Check sheet for the modelled part. Datum: model origin and axes. Units: mm. Face numbers are marked on the shaded views. A direction names the side the tool comes from. Give positions to 0.01 mm unless a question says otherwise; leave off trailing zeros. Loops run counter-clockwise (first coordinate to the right, second up) from the corner with the lowest first, then second, coordinate; pieces in that order, holes last. Notation, with made-up numbers: M 25.25,3.25 L 54.25,3.25 A23 ccw 54.25,28.25 Z; hole C 52,67 d9. An arc over 180 degrees is marked long. One line per question, with ' | ' between items. Start each with the question number.
from build123d import *

# Parameters (mm, degrees)
BOSS_EXTRUDE1_DEPTH = 22
SKETCH3_R           = 26.2
CUT_EXTRUDE1_DEPTH  = 10
BOSS_EXTRUDE2_START = -3
SKETCH4_R           = 7
BOSS_EXTRUDE2_DEPTH = 3
SKETCH5_R           = 1.8
CUT_EXTRUDE2_DEPTH  = 5
SKETCH6_R           = 1.6
CUT_EXTRUDE3_DEPTH  = 119.253467405
SKETCH7_R           = 1.6
CUT_EXTRUDE4_DEPTH  = 119.253467405


with BuildPart() as part:
    # Sketch2 → Boss-Extrude1 (new body)
    with BuildSketch(Plane.XY):
        with BuildLine():
            Line((81.411807591, -46.460279646), (18.828747548, 18.218624146))
            ThreePointArc((18.828747548, 18.218624146), (-18.218624146, 18.828747548), (-18.828747548, -18.218624146))
            Line((-18.828747548, -18.218624146), (43.754312495, -82.897527937))
            Line((43.754312495, -82.897527937), (55.216851555, -71.806418963))
            Line((55.216851555, -71.806418963), (53.478433221, -70.009782747))
            Line((53.478433221, -70.009782747), (68.210850196, -55.754752404))
            Line((68.210850196, -55.754752404), (69.94926853, -57.55138862))
            Line((69.94926853, -57.55138862), (81.411807591, -46.460279646))
        make_face()
        with BuildLine():
            Line((37.468734256, -8.236041156), (74.341698489, -46.343843882))
            Line((74.341698489, -46.343843882), (43.870748258, -75.827418835))
            Line((43.870748258, -75.827418835), (6.997784026, -37.719616109))
            Line((6.997784026, -37.719616109), (-15.235475115, -14.741787477))
            ThreePointArc((-15.235475115, -14.741787477), (-14.741787477, 15.235475115), (15.235475115, 14.741787477))
            Line((15.235475115, 14.741787477), (37.468734256, -8.236041156))
        make_face(mode=Mode.SUBTRACT)
    extrude(amount=BOSS_EXTRUDE1_DEPTH)

    # Sketch3 → Cut-Extrude1 (cut)
    with BuildSketch(Plane(origin=(0, 0, 0), x_dir=(-1, 0, 0), z_dir=(0, 0, -1))):
        Circle(SKETCH3_R)
    extrude(amount=-CUT_EXTRUDE1_DEPTH, mode=Mode.SUBTRACT)

    # Sketch4 → Boss-Extrude2 (add)
    with BuildSketch(Plane.XY.offset(22).offset(BOSS_EXTRUDE2_START)):
        with BuildLine():
            Line((43.870748258, -75.827418835), (74.341698489, -46.343843882))
            Line((74.341698489, -46.343843882), (15.235475115, 14.741787477))
            ThreePointArc((15.235475115, 14.741787477), (14.741787477, -15.235475115), (-15.235475115, -14.741787477))
            Line((-15.235475115, -14.741787477), (43.870748258, -75.827418835))
        make_face()
        with Locations((40.961727216, -42.477303154)):
            Circle(SKETCH4_R, mode=Mode.SUBTRACT)
        with BuildLine():
            Line((24.96542229, -18.72640467), (27.045904207, -20.887791955))
            ThreePointArc((27.045904207, -20.887791955), (27.325259938, -21.600355505), (27.018935751, -22.301748355))
            Line((27.018935751, -22.301748355), (21.255236326, -27.849700134))
            ThreePointArc((21.255236326, -27.849700134), (20.542672775, -28.129055865), (19.841279925, -27.822731678))
            Line((19.841279925, -27.822731678), (17.760798008, -25.661344393))
            ThreePointArc((17.760798008, -25.661344393), (17.481442277, -24.948780843), (17.787766464, -24.247387993))
            Line((17.787766464, -24.247387993), (23.551465889, -18.699436214))
            ThreePointArc((23.551465889, -18.699436214), (24.264029439, -18.420080483), (24.96542229, -18.72640467))
        make_face(mode=Mode.SUBTRACT)
    extrude(amount=BOSS_EXTRUDE2_DEPTH)

    # Sketch5 → Cut-Extrude2 (cut)
    with BuildSketch(Plane(origin=(62.583060043, -64.678903792, 0), x_dir=(0.7186544865731441, 0.6953673338087509, 0), z_dir=(0.6953673338087509, -0.7186544865731441, 0))):
        with Locations((15.5, 11.5)):
            Circle(SKETCH5_R)
        with Locations((-15.5, 11.5)):
            Circle(SKETCH5_R)
    extrude(amount=-CUT_EXTRUDE2_DEPTH, mode=Mode.SUBTRACT)

    # Sketch6 → Cut-Extrude3 (cut, through all)
    with BuildSketch(Plane.XY.offset(22)):
        with Locations((77.87675304, -46.402061764)):
            Circle(SKETCH6_R)
        with Locations((43.812530376, -79.362473386)):
            Circle(SKETCH6_R)
    extrude(amount=-CUT_EXTRUDE3_DEPTH, mode=Mode.SUBTRACT)

    # Sketch7 → Cut-Extrude4 (cut, through all)
    with BuildSketch(Plane.XY.offset(22)):
        with Locations((-16.461094787, 17.012360299)):
            Circle(SKETCH7_R)
        with Locations((17.012360299, 16.461094787)):
            Circle(SKETCH7_R)
        with Locations((16.461094787, -17.012360299)):
            Circle(SKETCH7_R)
        with Locations((-17.012360299, -16.461094787)):
            Circle(SKETCH7_R)
    extrude(amount=-CUT_EXTRUDE4_DEPTH, mode=Mode.SUBTRACT)


solid = part.part
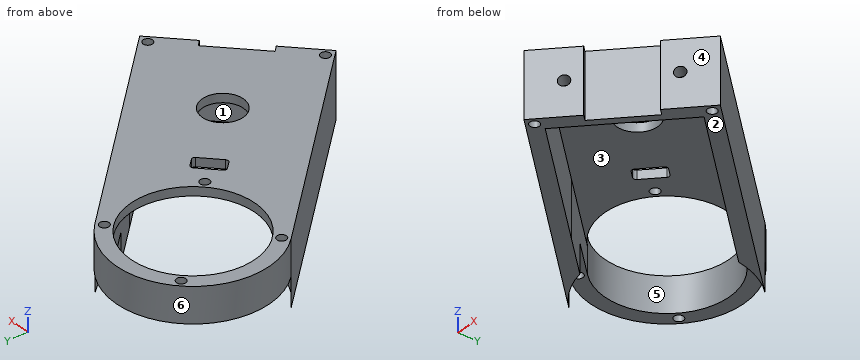
Q1. Depth check by flat-ended pin: P1, Ø5, axis at y = -59.5, z = 5.5, coming from the -X side; P2, Ø2.5, axis at x = -16.46, y = 17.01, coming from the -Z side; P3, Ø3, axis at x = 38.5, z = 7, coming from the +Y side; P4, Ø1.5, axis at y = -5, z = 9.5, coming from the -X side. Enter the tip coordinate at first touch or a pass-through.
Q2. Material ranges on probe 1 along Y at (x, z) = (16.5, 14.75); probe 2 along X at (y, z) = (3.5, 12); probe 3 along Y at (x, z) = (65.5, 7.75), recorded low to high. Write a range as from..to.
Q3. Access from +Z, -Z, +X, -X, +Y, -Y to the whole of each face (thin tool, end or side, straight path). Record for the marked faces 1 and 2.
Q4. Draft check along Y on the marked faces 3, 4, 5 and 6. Enter one of: released by +Y, released by -Y, zero draft, split by the parting line, or undercut.
Q5. Cross-section at A-A (x = 0). Record the cut outline in (y, z), and give its area (3 significant figures).
Q6. Cross-section at C-C (z = 1.5). Record the cut outline in (x, y), and give its area (3 significant figures).
Q7. Cross-section at B-B (y = 0). Record the cut outline in (x, z).
Q8. Cross-section at D-D (y = -33). Record the cut outline in (x, z), and give its area (3 significant figures).
Solved:
1) P1: stops at x = 18.7 | P2: passes through | P3: stops at y = -0.56 | P4: stops at x = -25.82
2) probe 1: y = -54.73..-47.54, 13.43..14.95, 17.98..20.35 | probe 2: x = -25.97..-20.91, 26.11..33.07 | probe 3: y = -58.38..-54.9, -37.21..-30.02
3) face 1: -Z | face 2: -Z, +X, -X, +Y, -Y
4) face 3: undercut | face 4: released by -Y | face 5: undercut | face 6: split by the parting line
5) outline: M -37.68,0 L -30.49,0 L -30.49,19 L -21.2,19 L -21.2,22 L -37.68,22 Z; M 21.2,10 L 26.2,10 L 26.2,22 L 21.2,22 Z | area: 246 mm²
6) outline: M -18.83,-18.22 L 43.75,-82.9 L 55.22,-71.81 L 53.48,-70.01 L 68.21,-55.75 L 69.95,-57.55 L 81.41,-46.46 L 18.83,18.22 A26.2 cw 25.94,3.68 L 74.34,-46.34 L 43.87,-75.83 L -4.53,-25.81 A26.2 cw Z; hole C 43.81,-79.36 d3.2; hole C 77.88,-46.4 d3.2 | area: 940 mm²
7) outline: M -26.2,10 L -21.2,10 L -21.2,22 L -26.2,22 Z; M 21.2,19 L 29.5,19 L 29.5,0 L 36.46,0 L 36.46,22 L 21.2,22 Z
8) outline: M -4.53,0 L 2.43,0 L 2.43,19 L 61.43,19 L 61.43,0 L 68.39,0 L 68.39,22 L -4.53,22 Z | area: 483 mm²
